Check sheet for the modelled part. Datum: model origin and axes. Units: mm. Give positions to 0.01 mm unless a question says otherwise; leave off trailing zeros. Write each question's results on one line, items separated by ' | '.
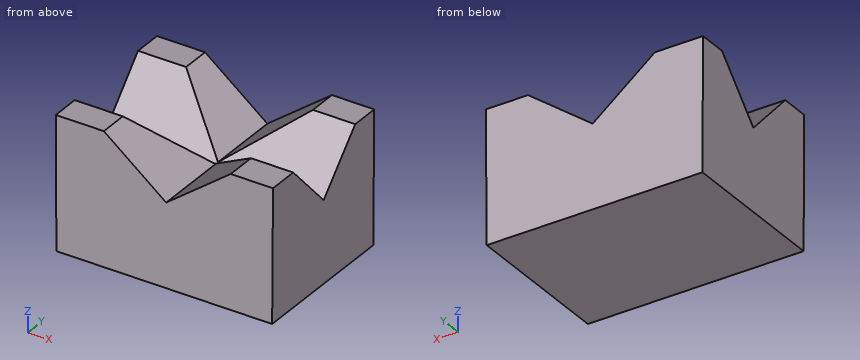
from build123d import *

# Parameters (mm, degrees)
F0_W   = 82.996623
F0_H   = 59.103658
F2_W   = 18.487399
F2_H   = 11.092441
F2_W_2 = 16.268921
F2_H_2 = 11.831935
F2_H_3 = 11.092439


with BuildPart() as f3:
    # F0 (on Top) → F3 section 0
    with BuildSketch(Plane.XY):
        with Locations((11.946483, -10.531769)):
            Rectangle(F0_W, F0_H)
    # F2 (on offset) → F3 section 1
    with BuildSketch(Plane.XY.offset(50.8)):
        with Locations((-20.656906, 13.695306)):
            Rectangle(F2_W, F2_H)
    loft()

    # F0 (on Top) → F4 section 0
    with BuildSketch(Plane.XY):
        with Locations((11.946483, -10.531769)):
            Rectangle(F0_W, F0_H)
    # F2 (on offset) → F4 section 1
    with BuildSketch(Plane.XY.offset(50.8)):
        with Locations((45.527997, -34.00219)):
            Rectangle(F2_W_2, F2_H_2)
    loft()

    # F0 (on Top) → F5 section 0
    with BuildSketch(Plane.XY):
        with Locations((11.946483, -10.531769)):
            Rectangle(F0_W, F0_H)
    # F2 (on offset) → F5 section 1
    with BuildSketch(Plane.XY.offset(50.8)):
        with Locations((-20.656906, -34.371938)):
            Rectangle(F2_W, F2_H_3)
    loft()

    # F0 (on Top) → F6 section 0
    with BuildSketch(Plane.XY):
        with Locations((11.946483, -10.531769)):
            Rectangle(F0_W, F0_H)
    # F2 (on offset) → F6 section 1
    with BuildSketch(Plane.XY.offset(50.8)):
        with Locations((45.527997, 13.695306)):
            Rectangle(F2_W_2, F2_H)
    loft()


solid = f3.part
1. Gauge pin test, flat ends, axial feed: pin 1 Ø4 at (y, z) = (-1, 8.5) entering from -X; pin 2 Ø6 at (y, z) = (-20.5, 26) entering from +X; pin 3 Ø5 at (y, z) = (-18.5, 24.5) entering from -X. Record the tip position at first contact, or that the pin passes through.
Verdict:
pin 1: stops at x = -29.62 | pin 2: stops at x = 53.57 | pin 3: stops at x = -29.74
2. Section check A-A on z = 43.5. Give the number of separate pieces and of enclosed holes in the cut face, then the cut area to 3 significant figures.
Verdict:
separate pieces: 4 | enclosed holes: 0 | area: 1,950 mm^2
3. Material ranges on probe 1 along Y at (x, z) = (-17.5, 40.5); probe 2 along Y at (x, z) = (-1, 39); probe 3 along X at (y, z) = (-25, 34.5), recorded low to high. Write a range as from..to.
Verdict:
probe 1: y = -39.95..-19.12, -1.63..19.2 | probe 2: y = -39.96..-17.71, -3.05..19.19 | probe 3: x = -29.79..9.4, 15.91..53.59
